Check sheet for the drawn part. Datum: minimum x, y, z corner. Units: mm. Give positions to 0.01 mm unless a question says otherwise; leave off trailing zeros. Loops run counter-clockwise (first coordinate to the right, second up) from the corner with the lowest first, then second, coordinate; pieces in that order, holes last.
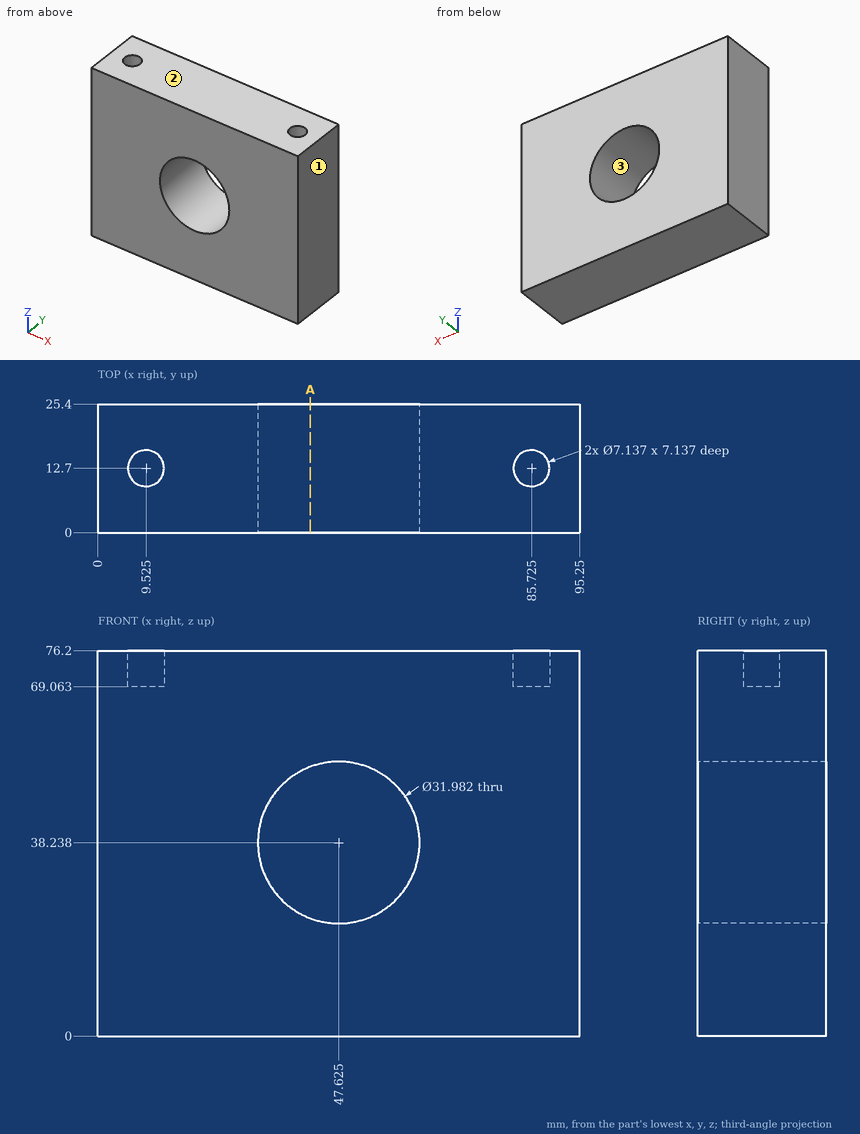
(1) Section check A-A on x = 42. Record the boundary of the cut face in (y, z), plus the area to 4 significant figures.
(2) Release check for a two-part mould opening along X. For the marked faces 1, 2 and 3 record: pulls with the +X half, pulls with the -X half, needs draft (parallel to the pull), parting line crosses it, or undercut.
(3) Material ranges on line 1 (Z direction, x = 85, y = 14.5); line 2 (Z direction, x = 57, y = 2.75) (1 decimal); line 3 (Z direction, x = 59.5, y = 14.75), recorded low to high.
Computed values:
1. outline: (0, 0) - (25.4, 0) - (25.4, 23.27) - (0, 23.27) - close; (0, 53.21) - (25.4, 53.21) - (25.4, 76.2) - (0, 76.2) - close
1. area: 1,175 mm2
2. face 1: pulls with the +X half
2. face 2: needs draft
2. face 3: undercut
3. line 1: z = 0 to 69.06
3. line 2: z = 0 to 25.3, 51.2 to 76.2
3. line 3: z = 0 to 27.53, 48.95 to 76.2
